The listing builds one solid part. Answer for the finished solid, in the listing's coordinates (mm). A direction names the side the tool comes from. Coordinates: 2 decimals unless noted, no trailing zeros. Order: outer loops, then holes, each group sorted by start corner. A loop starts at its lowest first (then second) coordinate and runs counter-clockwise, first axis right, second up. Notation, with made-up numbers: (64, 15.5) - (102, 15.5) arc R36 cw to (102, 49.5) - close; hole circle Ø3 at (38, 45.5). An arc over 180 degrees is marked (long way). Use one line per item in the form item = value. Start each with the question number.
Item 1: Consider line 1 along Z through (x, y) = (51.5, -47.5); line 2 along X through (y, z) = (27, 78); line 3 along Y through (x, z) = (11.5, 132.5). Determine where each line is inside the solid, lowest interval first. Write a range as [from, to].
Item 2: This flat-tipped pin is pushed along its axis until it touches: pin 1 Ø12 at (x, z) = (49.5, 144.5) entering from -Y. Where does it stop, or does it pass through?
Item 3: Section C-C, the plane x = -70 is taken. Write down the section's boundary in (y, z).
Item 4: A tool of negligible diameter and unlimited length cuts with its end or side. For faces 1 (the flat face through (-10, 77.112, 142)), 2 (the flat face through (-10, 59.332, 143)), from which of +Z, -Z, +X, -X, +Y, -Y can it reach the whole face along a straight path? Write none if from no direction.
Item 5: The mould has two halves that part along Z. Classify faces 3 (the flat face through (-10, -20, 270.764)), 4 (the flat face through (-10, -11, 288.544)), 5 (the flat face through (-10, -20, 17.78)), 6 (the flat face through (-81, -100.774, 133)): released by +Z, released by -Z, zero draft, split by the parting line, or undercut.
Item 6: Section A-A, the plane y = -24 is taken. Write down the section's boundary in (x, z), and give its area (3 significant figures).
Item 7: Section B-B, the plane z = 204.5 is taken. Write down the section's boundary in (x, y), and give its area (3 significant figures).
from build123d import *

# Parameters (mm, degrees)
F0_W     = 171.114452
F0_H     = 177.886084
F1_DEPTH = 288.544
F2_T     = -17.78
F3_SIZE  = 5.08


with BuildPart() as f1:
    # F0 (on Top) → F1 (new body)
    with BuildSketch(Plane.XY):
        with Locations((-8.802969, -11.831455)):
            Rectangle(F0_W, F0_H)
    extrude(amount=F1_DEPTH)

    # F2
    f2_openings = [f1.faces().sort_by_distance(p)[0] for p in [
        (-8.802969, -100.774497, 144.272),
    ]]
    offset(amount=F2_T, openings=f2_openings)

    # F3
    f3_edges = [f1.edges().sort_by_distance(p)[0] for p in [
        (-8.802969, -100.774497, 288.544),
        (76.754257, -11.831455, 288.544),
        (-8.802969, 77.111587, 288.544),
        (-94.360195, -11.831455, 288.544),
        (-94.360195, 77.111587, 144.272),
        (76.754257, 77.111587, 144.272),
        (76.754257, -100.774497, 144.272),
        (-94.360195, -100.774497, 144.272),
        (-94.360195, -11.831455, 0),
        (-8.802969, -100.774497, 0),
        (76.754257, -11.831455, 0),
        (-8.802969, 77.111587, 0),
    ]]
    chamfer(f3_edges, length=F3_SIZE)


solid = f1.part
Response:
q1.line_1 = [0, 17.78], [270.76, 288.54]
q1.line_2 = [-94.36, -76.58], [58.97, 76.75]
q1.line_3 = [59.33, 77.11]
q2.pin_1 = 59.33
q3.outline = (-100.77, 5.08) - (-95.69, 0) - (72.03, 0) - (77.11, 5.08) - (77.11, 283.46) - (72.03, 288.54) - (-95.69, 288.54) - (-100.77, 283.46) - (-100.77, 270.76) - (59.33, 270.76) - (59.33, 17.78) - (-100.77, 17.78) - close
q4.face_1 = +Z, -Z, +X, -X, +Y
q4.face_2 = -Y
q5.face_3 = undercut
q5.face_4 = released by +Z
q5.face_5 = undercut
q5.face_6 = zero draft
q6.outline = (-94.36, 5.08) - (-89.28, 0) - (71.67, 0) - (76.75, 5.08) - (76.75, 283.46) - (71.67, 288.54) - (-89.28, 288.54) - (-94.36, 283.46) - close; hole (-76.58, 17.78) - (58.97, 17.78) - (58.97, 270.76) - (-76.58, 270.76) - close
q6.area = 15,000 mm2
q7.outline = (-94.36, -95.69) - (-89.28, -100.77) - (-76.58, -100.77) - (-76.58, 59.33) - (58.97, 59.33) - (58.97, -100.77) - (71.67, -100.77) - (76.75, -95.69) - (76.75, 72.03) - (71.67, 77.11) - (-89.28, 77.11) - (-94.36, 72.03) - close
q7.area = 8,680 mm2
